from build123d import *

# Parameters (mm, degrees)
SKETCH1_R           = 12.827
BOSS_EXTRUDE1_DEPTH = 20.32
SKETCH2_R           = 12.827
SKETCH2_R_2         = 11.43
SKETCH2_R_3         = 6.35
BOSS_EXTRUDE2_DEPTH = 2.54


with BuildPart() as part:
    # Sketch1 → Boss-Extrude1 (new body)
    with BuildSketch(Plane.XY):
        Circle(SKETCH1_R)
    extrude(amount=BOSS_EXTRUDE1_DEPTH)

    # Sketch2 → Boss-Extrude2 (add)
    # profile 1 of 2: a face of its own
    with BuildSketch(Plane.XY.offset(20.32)):
        Circle(SKETCH2_R)
        Circle(SKETCH2_R_2, mode=Mode.SUBTRACT)
    # profile 2 of 2: a face of its own
    with BuildSketch(Plane.XY.offset(20.32)):
        Circle(SKETCH2_R_3)
    extrude(amount=BOSS_EXTRUDE2_DEPTH)


solid = part.part
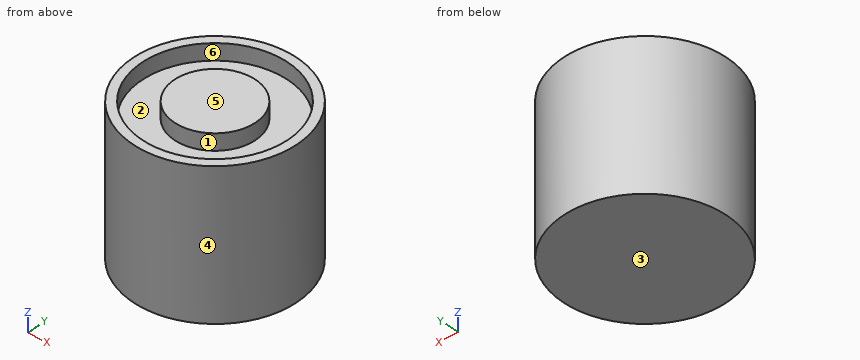
CAD build for the part. Positions are in the model's coordinates, mm. Face numbers are marked on the shaded views. A direction names the side the tool comes from. Round coordinates to 2 decimals unless told otherwise and drop trailing zeros. Loops run counter-clockwise (first coordinate to the right, second up) from the corner with the lowest first, then second, coordinate; pieces in that order, holes last.
(1) Which spindle directions (+Z, -Z, +X, -X, +Y, -Y) get a long thin tool onto all of the face, cutting with end or side? Do the marked faces 5 and 6. Say none if no direction does.
(2) Drop flat-ended pins along their axis: pin 1 (3 mm diameter, centred on x = 1, z = 10.5, fed in from +Y); pin 2 (3 mm diameter, centred on x = 8.5, z = 4.5, fed in from -Y); pin 3 (1.5 mm diameter, centred on y = -8.5, z = 4, fed in from +X); pin 4 (6 mm diameter, centred on x = -7.5, z = 15, fed in from +Y). Give the stop position or say it passes through.
(3) Cut at C-C (z = 8). Give the cut face in (x, y).
(4) Wall check: line 1 along Y through (x, z) = (0, 21.65); line 2 along X through (y, z) = (1.5, 20.5); line 3 along Z through (x, y) = (-7.5, 4.25). Give the ranges that are in metal, low to high.
(5) Two-plate mould, pull along X, no slides. Class the marked faces 1, 2, 3 and 4: +X half, -X half, draft (parallel to the pull), parting line (faces both ways), or undercut.
(6) Cut at A-A (y = 0). Give the cut face in (x, z), plus the area to 3 significant figures.
(7) Cut at D-D (x = -7). Give the cut face in (y, z).
Findings below:
1. face 5: +Z, +X, -X, +Y, -Y
1. face 6: +Z
2. pin 1: stops at y = 12.83
2. pin 2: stops at y = -10.75
2. pin 3: stops at x = 10.22
2. pin 4: stops at y = 12.01
3. outline: circle Ø25.65 at (0, 0)
4. line 1: y = -12.83 to -11.43, -6.35 to 6.35, 11.43 to 12.83
4. line 2: x = -12.74 to -11.33, -6.17 to 6.17, 11.33 to 12.74
4. line 3: z = 0 to 20.32
5. face 1: undercut
5. face 2: undercut
5. face 3: draft
5. face 4: parting line
6. outline: (-12.83, 0) - (12.83, 0) - (12.83, 22.86) - (11.43, 22.86) - (11.43, 20.32) - (6.35, 20.32) - (6.35, 22.86) - (-6.35, 22.86) - (-6.35, 20.32) - (-11.43, 20.32) - (-11.43, 22.86) - (-12.83, 22.86) - close
6. area: 561 mm2
7. outline: (-10.75, 0) - (10.75, 0) - (10.75, 22.86) - (9.04, 22.86) - (9.04, 20.32) - (-9.04, 20.32) - (-9.04, 22.86) - (-10.75, 22.86) - close
